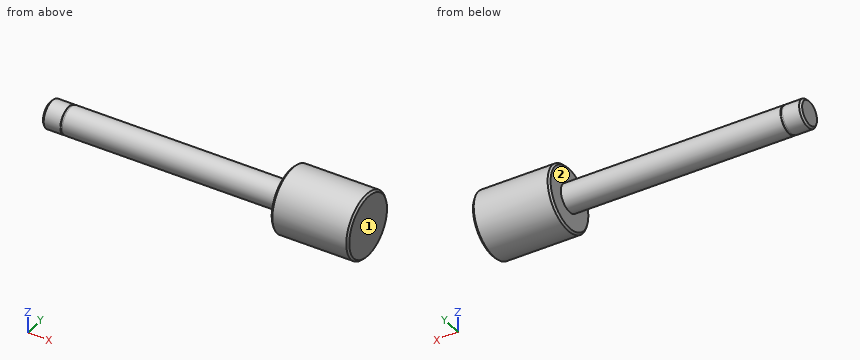
```python
from build123d import *

# Parameters (mm, degrees)
CHANFREIN1_SIZE = 1
ESQUISSE2_W     = 1.1
ESQUISSE2_H     = 8.504088504


with BuildPart() as part:
    # Esquisse1 → Révolution1 (revolve)
    with BuildSketch(Plane.XY, mode=Mode.PRIVATE) as r_volution1_sk:
        Polygon((-86, 0), (-86, 7.5), (44, 7.5), (44, 17.5), (86, 17.5), (86, 0), align=None)
    revolve(r_volution1_sk.sketch.rotate(Axis((-86, 0, 0), (1, 0, 0)), 90), axis=Axis((-86, 0, 0), (1, 0, 0)))  # turned: the seam where the file's is

    # Chanfrein1
    chanfrein1_edges = [part.edges().sort_by_distance(p)[0] for p in [
        (86, 0, -17.5),
        (44, 0, -17.5),
        (-86, 0, -7.5),
    ]]
    chamfer(chanfrein1_edges, length=CHANFREIN1_SIZE)

    # Esquisse2 → Enlèvement de matière-Révolution1 (revolve, cut)
    with BuildSketch(Plane.XY, mode=Mode.PRIVATE) as enl_vement_de_mati_re_r_volution1_sk:
        with Locations((-75.45, 11.402044252)):
            Rectangle(ESQUISSE2_W, ESQUISSE2_H)
    revolve(enl_vement_de_mati_re_r_volution1_sk.sketch.rotate(Axis((0, 0, 0), (-1, 0, 0)), 270), axis=Axis((0, 0, 0), (-1, 0, 0)), mode=Mode.SUBTRACT)  # turned: the seam where the file's is


solid = part.part
```
CAD build for the part. Positions are in the model's coordinates, mm. Face numbers are marked on the shaded views. A direction names the side the tool comes from. Coordinates: 2 decimals unless noted, no trailing zeros. Order: outer loops, then holes, each group sorted by start corner. A loop starts at its lowest first (then second) coordinate and runs counter-clockwise, first axis right, second up.
(1) Saw through at C-C, the plane x = 50. Write the cut outline in (y, z), and give its area (3 significant figures).
Solution:
outline: circle Ø35 at (0, 0)
area: 962 mm2
(2) Drill centre lines: L1, parallel to X at y = 15, z = -1; L2, parallel to Y at x = 14, z = 0.5; L3, parallel to Y at x = 73, z = 6. Where is each one in solid material? Low to high.
Solution:
L1: x = 44 to 86
L2: y = -7.48 to 7.48
L3: y = -16.44 to 16.44
(3) Pin check, flat tips, straight feed: pin 1 Ø4 at (x, z) = (-15, 5) entering from -Y; pin 2 Ø1.5 at (x, y) = (30.5, 7) entering from -Z; pin 3 Ø8 at (y, z) = (10.5, -3) entering from -X. Stop position of each tip, or through.
Solution:
pin 1: stops at y = -6.87
pin 2: stops at z = -4.15
pin 3: stops at x = -85.58
(4) Saw through at D-D, the plane x = 4.5. Write the cut outline in (y, z), and give its area (3 significant figures).
Solution:
outline: circle Ø15 at (0, 0)
area: 177 mm2
(5) Which spindle directions (+Z, -Z, +X, -X, +Y, -Y) get a long thin tool onto all of the face, cutting with end or side? Do the marked faces 1 and 2. Say none if no direction does.
Solution:
face 1: +Z, -Z, +X, +Y, -Y
face 2: -X
(6) Saw through at A-A, the plane y = 0. Write the cut outline in (x, z), and give its area (3 significant figures).
Solution:
outline: (-86, -6.5) - (-85, -7.5) - (-76, -7.5) - (-76, -7.15) - (-74.9, -7.15) - (-74.9, -7.5) - (44, -7.5) - (44, -16.5) - (45, -17.5) - (85, -17.5) - (86, -16.5) - (86, 16.5) - (85, 17.5) - (45, 17.5) - (44, 16.5) - (44, 7.5) - (-74.9, 7.5) - (-74.9, 7.15) - (-76, 7.15) - (-76, 7.5) - (-85, 7.5) - (-86, 6.5) - close
area: 3,420 mm2
